Autodesk Inventor part; units mm, degrees
ref_plane "YZ Plane" through (0, 0, 0) normal (1, 0, 0) x (0, 1, 0)
ref_plane "XZ Plane" through (0, 0, 0) normal (0, 1, 0) x (-1, 0, 0)
ref_plane "XY Plane" through (0, 0, 0) normal (0, 0, 1) x (1, 0, 0)
sketch "Sketch1" plane through (0, 0, 0) normal (1, 0, 0) x (0, 1, 0)
  circle A0 centre (0, 0) radius 17.78
  dimension "d0" = 35.56
extrude "Extrusion1" add sketch "Sketch1" along normal blind 1.27
sketch "Sketch2" plane through (1.27, 0, 0) normal (1, 0, 0) x (0, 0, -1)
  circle A0 centre (0, 0) radius 17.78
  circle A1 centre (0, 0) radius 16.51
  dimension "d3" = 35.56
  dimension "d4" = 33.02
extrude "Extrusion2" add sketch "Sketch2" along normal blind 9.652
sketch "Sketch3" plane through (10.922, 0, 0) normal (1, 0, 0) x (0, 0, -1)
  line L0 (-20.45, -20.45) -> (20.45, -20.45)
  line L1 (20.45, -20.45) -> (20.45, 20.45)
  line L2 (20.45, 20.45) -> (-20.45, 20.45)
  line L3 (-20.45, 20.45) -> (-20.45, -20.45)
  line L4 (-20.45, -20.45) -> (20.45, 20.45) construction
  line L5 (20.45, -20.45) -> (-20.45, 20.45) construction
  point P0 (0, 0)
  dimension "d7" = 40.9
  dimension "d8" = 40.9
extrude "Extrusion3" add sketch "Sketch3" along normal blind 1.27
sketch "Sketch4" plane through (12.192, 0, 0) normal (1, 0, 0) x (0, 0, -1)
  circle A0 centre (0, 0) radius 16.51
  line L0 (-20.45, 20.45) -> (-20.45, -20.45)
  line L1 (20.45, -20.45) -> (20.45, 20.45)
  line L2 (-20.45, -20.45) -> (20.45, -20.45)
  line L3 (20.45, 20.45) -> (-20.45, 20.45)
  line L4 (-16.7742, -16.7449) -> (16.7742, -16.745)
  line L5 (16.7742, -16.745) -> (16.7742, 16.745)
  line L6 (16.7742, 16.745) -> (-16.7742, 16.7449)
  line L7 (-16.7742, 16.7449) -> (-16.7742, -16.7449)
  line L8 (-16.7742, -16.7449) -> (16.7742, 16.745) construction
  line L9 (16.7742, -16.745) -> (-16.7742, 16.7449) construction
  circle A1 centre (-16.7742, -16.7449) radius 1.6262
  circle A2 centre (16.7687, -16.8222) radius 1.6262
  circle A3 centre (16.6447, 16.6573) radius 1.6262
  circle A4 centre (-16.5868, 16.4713) radius 1.6262
  dimension "d18" = 33.02
  dimension "d25" = 40.9
  dimension "d32" = 33.4899
  dimension "d33" = 33.5483
  dimension "d34" = 3.2524
  dimension "d35" = 3.2524
  dimension "d36" = 3.2524
  dimension "d37" = 3.2524
extrude "Extrusion4" cut sketch "Sketch4" against normal blind 3.2524 contours A0 | L7 A1 L4 | L4 A1 L7 | A2 L5 L4 | L4 L5 A2 | A4 L6 L7 | L7 L6 A4 | A3 L6 L5 | L5 L6 A3
fillet "Fillet1" radius 1.778 1 edges at (10.922, 0, 17.78)
sketch "Sketch5" plane through (0, 0, 0) normal (-1, 0, 0) x (0, 0, 1)
  point P0 (0, 0)
equation "\"d16\" = d35"
properties part number "MagnetCap"
Could you check a few things on this model? Use its own coordinates, in mm. A direction names the side the tool comes from. Give positions to 0.01 mm unless a question says otherwise; leave off trailing zeros. Write each loop counter-clockwise with the first axis right and the second up, starting at its lowest first coordinate (ties: lowest second). Pieces come first, ordered by that corner, then holes. Notation, with made-up numbers: (29, -34) -> (51, -34) arc R30 ccw to (51, 4) -> close; hole circle Ø4 at (36.5, 73.25). An arc over 180 degrees is marked (long way). Answer as a JSON object with one key per item and string values.
Q1. Suppose I cut it at C-C on z = -17. Count the separate pieces of the cut face and the enclosed holes in it, then the cut area to 3 significant figures.
Taken from the geometry:
{"separate pieces": "3", "enclosed holes": "0", "area": "162 mm²"}
Q2. We'd pull the mould along Y, two halves only. Please class faces 1 (the flat face through (12, 20.45, 0)), 2 (the flat face through (10.922, 18.3, 7.7)), 3 (the cylindrical face through (11.57, 18.03, -17.52)): released by +Y, released by -Y, zero draft, split by the parting line, or undercut.
Taken from the geometry:
{"face 1": "released by +Y", "face 2": "zero draft", "face 3": "undercut"}
Q3. Which directions (+Z, -Z, +X, -X, +Y, -Y) give clear straight access to the entire face, cutting with the end or side of a thin tool? Please do faces 4 (the cylindrical face through (6.655, -4.959, -15.748)), 5 (the flat face through (12, -20.45, 0)).
Taken from the geometry:
{"face 4": "+X", "face 5": "+Z, -Z, +X, -X, -Y"}
Q4. Please list where these lines run through material, in increasing order: L1, parallel to X at y = 2.5, z = -15.5; L2, parallel to Y at x = 4, z = -4.5; L3, parallel to Z at x = 5.5, y = 7.5.
Taken from the geometry:
{"L1": "x = 0 to 1.27", "L2": "y = -17.2 to -15.88, 15.88 to 17.2", "L3": "z = -16.12 to -14.71, 14.71 to 16.12"}
Q5. Will these pins go through, and if not, where does the flat tip stop? pin 1 Ø5 at (x, y) = (7.5, 4) entering from -Z; pin 2 Ø1 at (x, y) = (8, -15) entering from +Z; pin 3 Ø4 at (y, z) = (16.66, -16.64) entering from -X.
Taken from the geometry:
{"pin 1": "stops at z = -17.72", "pin 2": "stops at z = 10.29", "pin 3": "stops at x = 10.92"}
Q6. Suppose I cut it at A-A on y = 0. Write out the boundary of the cut face in (x, z), then the cut area to 3 significant figures.
Taken from the geometry:
{"outline": "(0, -17.78) -> (9.14, -17.78) arc R1.78 cw to (10.92, -19.56) -> (10.92, -20.45) -> (12.19, -20.45) -> (12.19, -16.51) -> (1.27, -16.51) -> (1.27, 16.51) -> (12.19, 16.51) -> (12.19, 20.45) -> (10.92, 20.45) -> (10.92, 19.56) arc R1.78 cw to (9.14, 17.78) -> (0, 17.78) -> close", "area": "81.0 mm²"}
